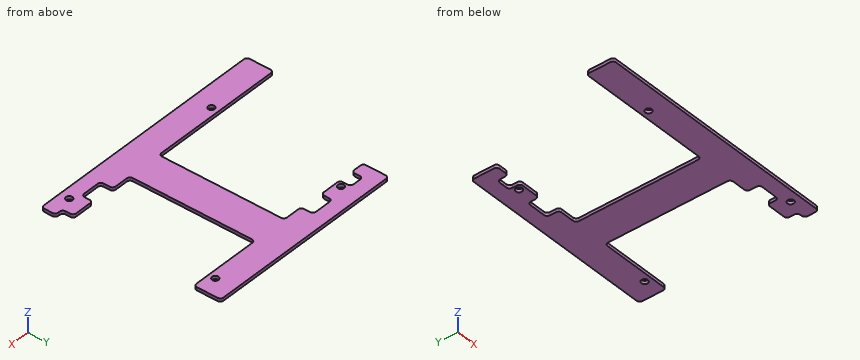
Autodesk Inventor part; units mm, degrees
ref_plane "YZ Plane" through (0, 0, 0) normal (1, 0, 0) x (0, 1, 0)
ref_plane "XZ Plane" through (0, 0, 0) normal (0, 1, 0) x (-1, 0, 0)
ref_plane "XY Plane" through (0, 0, 0) normal (0, 0, 1) x (1, 0, 0)
sketch "Sketch1" plane through (0, 0, 0) normal (0, 0, 1) x (1, 0, 0)
  circle A0 centre (-5.7295, 41.15) radius 1.0065
  circle A1 centre (-52.875, 41.15) radius 1.0065
  line L0 (-57.9354, 38.4) -> (-57.9354, 42.4)
  line L1 (-57.9354, 42.4) -> (-55.625, 42.4)
  line L2 (-55.625, 42.4) -> (-55.625, 38.4)
  line L3 (-55.625, 38.4) -> (-46.3947, 38.4)
  line L4 (-46.3947, 38.4) -> (-46.3947, 42.4)
  line L5 (-46.3947, 42.4) -> (-41.4006, 42.4)
  line L6 (-41.4006, 42.4) -> (-41.4006, 38.4)
  line L7 (-41.4006, 38.4) -> (0, 38.4)
  line L8 (0, 38.4) -> (0, 47.7)
  line L9 (0, 47.7) -> (-59.3371, 47.7)
  line L10 (-59.3371, 38.4) -> (-59.3371, 47.7)
  line L11 (-59.3371, 38.4) -> (-57.9354, 38.4)
  circle A2 centre (-56.5871, -2.75) radius 1.0065
  circle A3 centre (-7.1235, -6) radius 1.0065
  line L12 (-15.9365, -4) -> (-15.9365, 0)
  line L13 (-59.3371, 0) -> (-15.9365, 0)
  line L14 (-59.3371, 0) -> (-59.3371, -9.3)
  line L15 (-59.3371, -9.3) -> (0, -9.3)
  line L16 (0, -4) -> (0, -9.3)
  line L17 (0, -4) -> (-1.712, -4)
  line L18 (-1.712, -4) -> (-1.712, 0)
  line L19 (-10.9424, 0) -> (-1.712, 0)
  line L20 (-10.9424, 0) -> (-10.9424, -4)
  line L21 (-10.9424, -4) -> (-15.9365, -4)
  line L22 (-77.2, -9) -> (-65.2, -9)
  line L23 (-65.2, -9) -> (-65.2, 11)
  line L24 (-65.2, 11) -> (-77.2, 11)
  line L25 (-77.2, 11) -> (-77.2, -9)
  line L26 (-77.2, -9) -> (-0.2, -9)
  line L27 (-0.2, -9) -> (-0.2, -4.5)
  line L28 (-0.2, -4.5) -> (-2.7272, -4.5)
  line L29 (-2.7272, -4.5) -> (-2.7272, -1)
  line L30 (-2.7272, -1) -> (-9.9272, -1)
  line L31 (-9.9272, -1) -> (-9.9272, -4.5)
  line L32 (-9.9272, -4.5) -> (-17, -4.5)
  line L33 (-17, -4.5) -> (-17, -0.5)
  line L34 (-17, -0.5) -> (-77.2, -0.5)
  line L35 (-61.3371, -12.3) -> (-59.4157, -12.3)
  line L36 (-59.4157, -12.3) -> (-59.3371, -12.3)
  line L37 (-59.3371, 0) -> (-59.3371, -12.3)
  line L38 (-59.3371, 0) -> (-63.3371, 0)
  line L39 (-63.3371, 0) -> (-63.3371, -6.8)
  line L40 (-63.3371, -6.8) -> (-63.3371, -14.3)
  arc A4 (-61.3371, -12.3) -> (-63.3371, -14.3) centre (-61.3371, -14.3) ccw
  line L41 (-59.3371, 50.7) -> (-59.4157, 50.7)
  line L42 (-59.4157, 50.7) -> (-61.3371, 50.7)
  arc A5 (-63.3371, 52.7) -> (-61.3371, 50.7) centre (-61.3371, 52.7) ccw
  line L43 (-63.3371, 44.7) -> (-63.3371, 52.7)
  line L44 (-63.3371, 38.4) -> (-63.3371, 44.7)
  line L45 (-63.3371, 38.4) -> (-59.3371, 38.4)
  line L46 (-59.3371, 38.4) -> (-59.3371, 50.7)
  line L47 (-63.2, 47.5) -> (-0.2, 47.5)
  line L48 (-0.2, 47.5) -> (-0.2, 39)
  line L49 (-63.2, 39.4) -> (-63.2, 47.5)
  line L50 (6.5, 33.15) -> (-22.9, 33.15)
  line L51 (-34.4371, 33.15) -> (-63.8371, 33.15)
  line L52 (-34.4371, 5.25) -> (-63.8371, 5.25)
  line L53 (6.5, 5.25) -> (-22.9, 5.25)
  line L54 (-0.2, 39) -> (-40.4, 39)
  line L55 (-40.4, 39) -> (-40.4, 42.9)
  line L56 (-40.4, 42.9) -> (-47.5099, 42.9)
  line L57 (-47.5099, 42.9) -> (-47.5099, 39.4)
  line L58 (-47.5099, 39.4) -> (-54.5099, 39.4)
  line L59 (-54.5099, 39.4) -> (-54.5099, 42.9)
  line L60 (-54.5099, 42.9) -> (-59, 42.9)
  line L61 (-59, 42.9) -> (-59, 39.4)
  line L62 (-59, 39.4) -> (-63.2, 39.4)
  line L63 (-23.1685, -0.5) -> (-23.1685, 7.5)
  line L64 (-23.1685, 7.5) -> (-23.1685, 7.5)
  line L65 (-23.1685, 7.5) -> (-23.1685, 32.15)
  line L66 (-23.1685, 32.15) -> (-23.1685, 32.15)
  line L67 (-23.1685, 32.15) -> (-23.1685, 39)
  line L68 (-34.1685, 39) -> (-34.1685, 31)
  line L69 (-34.1685, 31) -> (-34.1685, 31)
  line L70 (-34.1685, 31) -> (-34.1685, -0.5)
  point P0 (0, 0)
  point P1 (-23.1685, 38.4)
  point P2 (-34.1685, 38.4)
  dimension "d0" = 12
  dimension "d1" = 20
  dimension "d3" = 0.3
  dimension "d4" = 8.5
  dimension "d5" = 0.5
  dimension "d6" = 4.5
  dimension "d7" = 0.5
  dimension "d8" = 8
  dimension "d9" = 1
  dimension "d10" = 7.2
  dimension "d11" = 1.0152
  dimension "d12" = 1.0152
  dimension "d14" = 0.2
  dimension "d15" = 77
  dimension "d16" = 60.2
  dimension "d17" = 1.0635
  dimension "d18" = 0.2
  dimension "d19" = 0.2
  dimension "d21" = 63
  dimension "d23" = 8.5
  dimension "d24" = 1
  dimension "d25" = 0.5
  dimension "d27" = 4.2
  dimension "d28" = 1.0646
  dimension "d29" = 1.1152
  dimension "d30" = 1.1152
  dimension "d31" = 7
  dimension "d32" = 8.1
  dimension "d33" = 1.0006
  dimension "d34" = 40.2
  dimension "d35" = 8
  dimension "d36" = 8
  dimension "d38" = 0.2685
  dimension "d39" = 0.2685
  dimension "d40" = 11
  dimension "d41" = 0.2685
  dimension "d42" = 0.2685
  dimension "d43" = 1
  dimension "d44" = 0.2685
extrude "Extrusion1" add sketch "Sketch1" along normal blind 1 contours L62 L49 L47 L10 | L10 L47 L48 L54 L55 L56 L57 L58 L59 L60 L61 L62 | L67 L7 L68 L54 | L67 L65 L63 L13 L70 L68 L7 | L13 L63 L34 L70 | L34 L33 L32 L31 L30 L29 L28 L27 L26 L14 | L14 L26 L40 L39 L34 | L39 L40 L26 L23 L34 | L23 L22 L25 L34
fillet "Fillet1" radius 1 26 edges at (-23.1685, 39, 0.5) (-23.1685, -0.5, 0.5) (-17, -0.5, 0.5) (-17, -4.5, 0.5) (-2.7272, -1, 0.5) (-9.9272, -1, 0.5) (-9.9272, -4.5, 0.5) (-2.7272, -4.5, 0.5) (-0.2, -4.5, 0.5) (-0.2, -9, 0.5) (-77.2, -9, 0.5) (-77.2, -0.5, 0.5) (-34.1685, -0.5, 0.5) (-34.1685, 39, 0.5) (-40.4, 39, 0.5) (-40.4, 42.9, 0.5) (-47.5099, 42.9, 0.5) (-47.5099, 39.4, 0.5) (-54.5099, 39.4, 0.5) (-54.5099, 42.9, 0.5) (-59, 42.9, 0.5) (-59, 39.4, 0.5) (-63.2, 39.4, 0.5) (-63.2, 47.5, 0.5) (-0.2, 47.5, 0.5) (-0.2, 39, 0.5)
equation "\"d11\" = d12"
equation "\"d23\" = d4"
equation "\"d25\" = d7"
equation "\"d30\" = d29"
equation "\"d36\" = d35"
equation "\"d39\" = d38"
equation "\"d41\" = d38"
equation "\"d42\" = d39"
equation "\"d44\" = d38"
properties part number "PCB_interface_v2"
The model under review builds one solid part; all positions refer to its coordinate system, in mm. Round coordinates to 2 decimals unless told otherwise and drop trailing zeros. Write each loop counter-clockwise with the first axis right and the second up, starting at its lowest first coordinate (ties: lowest second). Pieces come first, ordered by that corner, then holes. Notation, with made-up numbers: M -16,76.5 L 19,76.5 A19 cw 19,109.5 Z; hole C -19.5,47.5 d4. An arc over 180 degrees is marked long. Use a Markdown table: item, result. Add a question column.
Q1. We need section B-B, the plane y = 31.5. State the section outline as (x, z) points, plus the area to 3 significant figures.
Q2. Insertion check: pin 1 (0.5 mm diameter, centred on y = 41.5, z = 0.5, fed in from -X); pin 2 (1.6 mm diameter, centred on x = -5.73, y = 41.15, fed in from +Z); pin 3 (0.5 mm diameter, centred on y = 11.5, z = 0.5, fed in from -X). Each pin has a flat end and moves straight along its axis. Give the tip position at first contact, or say it passes through.
Q3. We need section D-D, the plane z = 0.55. Count the separate pieces of the cut face and the enclosed holes in it, plus the area to 3 significant figures.
Q4. To check wall thickness, follow line 1 (Y direction, x = -13.5, z = 0.35); line 2 (Y direction, x = -8.5, z = 0.1); line 3 (Y direction, x = -6, z = 0.6). State the ranges of each line that lie inside material, in increasing order.
Q5. We need section C-C, the plane x = -68. State the section outline as (y, z) points.
Q6. We need section A-A, the plane x = -51. State the section outline as (y, z) points, plus the area to 3 significant figures.
Findings below:
| question | item | result |
|---|---|---|
| 1 | outline | M -34.17,0 L -23.17,0 L -23.17,1 L -34.17,1 Z |
| 1 | area | 11.0 mm² |
| 2 | pin 1 | stops at x = -63.2 |
| 2 | pin 2 | passes through |
| 2 | pin 3 | stops at x = -34.17 |
| 3 | separate pieces | 1 |
| 3 | enclosed holes | 4 |
| 3 | area | 1,520 mm² |
| 4 | line 1 | y = -9 to -4.5, 39 to 47.5 |
| 4 | line 2 | y = -9 to -1, 39 to 47.5 |
| 4 | line 3 | y = -9 to -1, 39 to 40.18, 42.12 to 47.5 |
| 5 | outline | M -9,0 L -0.5,0 L -0.5,1 L -9,1 Z |
| 6 | outline | M -9,0 L -0.5,0 L -0.5,1 L -9,1 Z; M 39.4,0 L 47.5,0 L 47.5,1 L 39.4,1 Z |
| 6 | area | 16.6 mm² |
